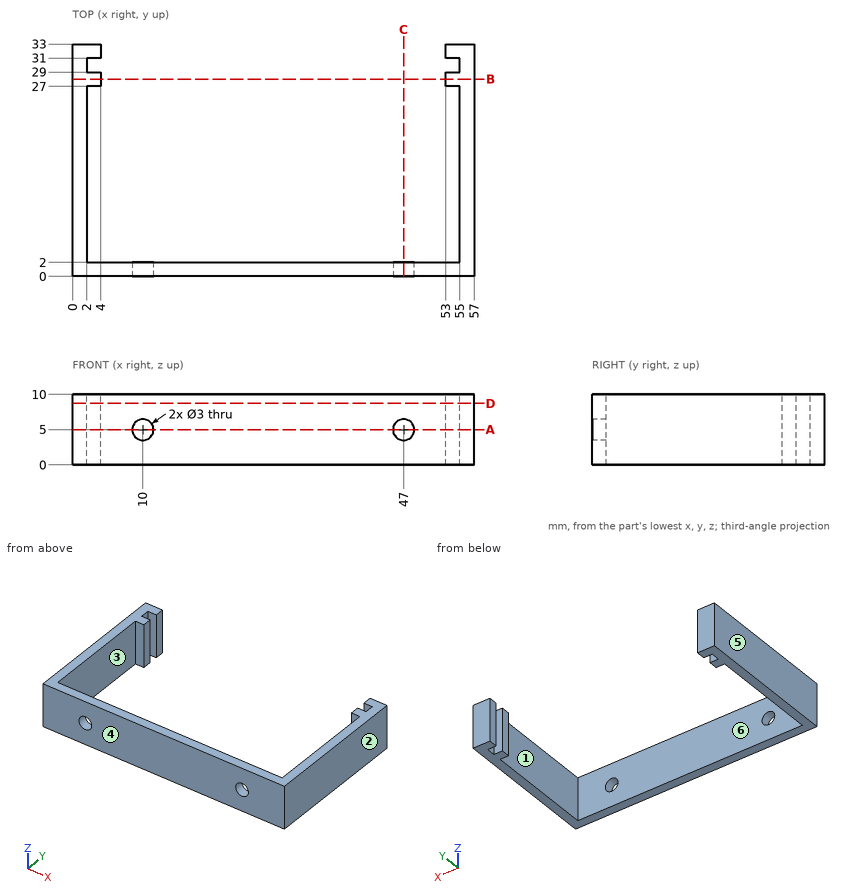
Answer from the drawing. Dimensions are ordinates in mm from the lowest x, y and z of the part. A direction names the side the tool comes from. Coordinates: 2 decimals unless noted, no trailing zeros. Write each loop counter-clockwise with the first axis right and the second up, starting at its lowest first coordinate (ties: lowest second). Pieces come first, ordered by that corner, then holes. Notation, with made-up numbers: M 20,59.5 L 78,59.5 A27 ccw 78,80.5 Z; hole C -5.5,3 d3. An arc over 180 degrees is marked long. Write item = value, one per line.
1. The part is cut by section B-B (y = 28). Determine the outline of the cut face in (x, z).
Solution:
outline = M 0,0 L 4,0 L 4,10 L 0,10 Z; M 53,0 L 57,0 L 57,10 L 53,10 Z
2. The part is cut by section D-D (z = 8.75). Determine the outline of the cut face in (x, y), then the cut area to 3 significant figures.
Solution:
outline = M 0,0 L 57,0 L 57,33 L 53,33 L 53,31 L 55,31 L 55,29 L 53,29 L 53,27 L 55,27 L 55,2 L 2,2 L 2,27 L 4,27 L 4,29 L 2,29 L 2,31 L 4,31 L 4,33 L 0,33 Z
area = 254 mm2
3. Straight lines are drawn through the part: line 1 (X direction, y = 28.5, z = 1.5); line 2 (Z direction, x = 10, y = 0.55); line 3 (X direction, y = 19, z = 3). For each, find the intervals that lie inside material, in ascending order. Write a range as from..to.
Solution:
line_1 = 0..4, 53..57
line_2 = 0..3.5, 6.5..10
line_3 = 0..2, 55..57
4. Determine the mould class of the marked faces 3, 4, 5 and 6 for opening direction X: released by +X, released by -X, zero draft, split by the parting line, or undercut.
Solution:
face_3 = undercut
face_4 = zero draft
face_5 = released by -X
face_6 = undercut
5. The part is cut by section C-C (x = 47). Determine the outline of the cut face in (y, z), then the cut area to 3 significant figures.
Solution:
outline = M 0,0 L 2,0 L 2,3.5 L 0,3.5 Z; M 0,6.5 L 2,6.5 L 2,10 L 0,10 Z
area = 14.0 mm2
6. For the marked faces 1 and 2, determine the directions among +Z, -Z, +X, -X, +Y, -Y from which every point of the face is accessible in a straight line to the end or side of a thin tool.
Solution:
face_1 = +Z, -Z
face_2 = +Z, -Z, +X, +Y, -Y
7. The part is cut by section A-A (z = 5). Determine the outline of the cut face in (x, y), then the cut area to 3 significant figures.
Solution:
outline = M 0,0 L 8.5,0 L 8.5,2 L 2,2 L 2,27 L 4,27 L 4,29 L 2,29 L 2,31 L 4,31 L 4,33 L 0,33 Z; M 11.5,0 L 45.5,0 L 45.5,2 L 11.5,2 Z; M 48.5,0 L 57,0 L 57,33 L 53,33 L 53,31 L 55,31 L 55,29 L 53,29 L 53,27 L 55,27 L 55,2 L 48.5,2 Z
area = 242 mm2
8. Flat-ended cylindrical pins translate along their axes: pin 1 (0.6 mm diameter, centred on y = 32, z = 4, fed in from -X); pin 2 (2.5 mm diameter, centred on x = 10, z = 5, fed in from -Y). Find the tip coordinate at first contact, or state that the pin passes through.
Solution:
pin_1 = 0
pin_2 = through
